CAD build for the part. Positions are in the model's coordinates, mm. A direction names the side the tool comes from. Give positions to 0.01 mm unless a question says otherwise; leave off trailing zeros. Loops run counter-clockwise (first coordinate to the right, second up) from the corner with the lowest first, then second, coordinate; pieces in that order, holes last. Notation, with made-up numbers: (-34.75, -26) - (-19.75, -26) arc R18 cw to (-19.75, 0) - close; hole circle Ø9 at (89.5, -28.75). An arc over 180 degrees is marked (long way). Return JSON: item names as keys, results as strings.
from build123d import *

# Parameters (mm, degrees)
SKETCH_1_R             = 1.55
SKETCH_1_W             = 8
SKETCH_1_H             = 3.5
EXTRUDE_1_DEPTH        = 2
EXTRUDE_START          = 2
EXTRUDE_2_DEPTH        = 2
FILLET_1_R             = 66.25
FILLET_4_R             = 1.5
SKETCH_7093_W          = 3
SKETCH_7093_H          = 15.5
SKETCH_7093_H_2        = 8.5
CUT_EXTRUDE_7585_DEPTH = 243.593574343
SKETCH_4_R             = 1.55
CUT_EXTRUDE_3_DEPTH    = 243.593574343
FILLET_5_R             = 3.5
SKETCH_8290_R          = 0.5
CUT_EXTRUDE_8728_DEPTH = 243.593574343


with BuildPart() as part:
    # 草图1 → 凸台-拉伸1 (new body)
    with BuildSketch(Plane.XY):
        with BuildLine():
            Line((155.184819061, -135.622927906), (110.023968778, -178.814555125))
            Line((110.023968778, -178.814555125), (45.146014647, -178.814555125))
            Line((45.146014647, -178.814555125), (22.125974708, -159.870216287))
            Line((22.125974708, -159.870216287), (-22.125974708, -159.870216287))
            Line((-22.125974708, -159.870216287), (-45.146014647, -178.814555125))
            Line((-45.146014647, -178.814555125), (-110.023968778, -178.814555125))
            Line((-110.023968778, -178.814555125), (-157.725302675, -148.011482983))
            Line((-157.725302675, -148.011482983), (-157.725302675, -39.583555807))
            Line((-157.725302675, -39.583555807), (-163.929854474, -22.461337388))
            Line((-163.929854474, -22.461337388), (-163.929854474, -5.84291361))
            Line((-163.929854474, -5.84291361), (-155.504077083, -3.600927376))
            Line((-155.504077083, -3.600927376), (-155.504077083, -0.25))
            Line((-155.504077083, -0.25), (-135.192862201, -0.25))
            Line((-135.192862201, -0.25), (-135.192862201, -5.85))
            Line((-135.192862201, -5.85), (-129.719705899, -10.576675864))
            Line((-129.719705899, -10.576675864), (-129.719705899, -18.798405758))
            Line((-129.719705899, -18.798405758), (-135.893457817, -19.398277466))
            Line((-135.893457817, -19.398277466), (-141.850432027, -24.52026455))
            Line((-141.850432027, -24.52026455), (-141.850432027, -87.17927527))
            ThreePointArc((-141.850432027, -87.17927527), (-143.273456416, -95.14794796), (-143.75, -103.228644035))
            ThreePointArc((-143.75, -103.228644035), (-106.74521716, -164.210638816), (-35.566620001, -159.54534708))
            Line((-35.566620001, -159.54534708), (-22.125974708, -150.134105928))
            Line((-22.125974708, -150.134105928), (22.125974708, -150.134105928))
            Line((22.125974708, -150.134105928), (35.566620001, -159.54534708))
            ThreePointArc((35.566620001, -159.54534708), (106.74521716, -164.210638816), (143.75, -103.228644035))
            ThreePointArc((143.75, -103.228644035), (143.461588771, -96.937907752), (142.598774895, -90.699951658))
            Line((142.598774895, -90.699951658), (142.966212817, -58.312660923))
            Line((142.966212817, -58.312660923), (131.782009345, -48.416521639))
            Line((131.782009345, -48.416521639), (120.077827626, -48.416521639))
            Line((120.077827626, -48.416521639), (114.577827626, -42.916521639))
            Line((114.577827626, -42.916521639), (114.577827626, -32.685002446))
            ThreePointArc((114.577827626, -32.685002446), (131.61274691, -32.289659724), (148.501080229, -30.024937097))
            ThreePointArc((148.501080229, -30.024937097), (150.418326561, -30.295579056), (151.770912833, -31.681072088))
            Line((151.770912833, -31.681072088), (155.01141709, -38.479630817))
            ThreePointArc((155.01141709, -38.479630817), (155.29338172, -39.526516509), (155.184819061, -40.605260155))
            Line((155.184819061, -40.605260155), (155.184819061, -135.622927906))
        make_face()
        with Locations((-133.806240002, -14.600927376)):
            Circle(SKETCH_1_R, mode=Mode.SUBTRACT)
        with Locations((120.182300402, -39.335)):
            Circle(SKETCH_1_R, mode=Mode.SUBTRACT)
        with Locations((149.25, -76.25)):
            Rectangle(SKETCH_1_W, SKETCH_1_H, mode=Mode.SUBTRACT)
        with Locations((-149.25, -76.25)):
            Rectangle(SKETCH_1_W, SKETCH_1_H, mode=Mode.SUBTRACT)
    extrude(amount=EXTRUDE_1_DEPTH)

    # 草图2 → 凸台-拉伸2 (add)
    with BuildSketch(Plane.XY.offset(EXTRUDE_START)):
        Polygon((155.184819061, -68.75), (158.934819061, -70.915063509), (158.934819061, -81.584936491), (155.184819061, -83.75), align=None)
        Polygon((-157.725302675, -68.75), (-157.725302675, -83.75), (-162.225302675, -81.886038969), (-162.225302675, -70.613961031), align=None)
    extrude(amount=-EXTRUDE_2_DEPTH)

    # 圆角1
    fillet_1_edges = [part.edges().sort_by_distance(p)[0] for p in [
        (-141.850432027, -87.17927527, 1),
        (142.598774895, -90.699951658, 1),
    ]]
    fillet(fillet_1_edges, radius=FILLET_1_R)

    # 圆角4
    fillet_4_edges = [part.edges().sort_by_distance(p)[0] for p in [
        (158.934819061, -81.584936491, 1),
        (158.934819061, -70.915063509, 1),
        (155.184819061, -68.75, 1),
        (155.184819061, -83.75, 1),
        (-162.225302675, -70.613961031, 1),
        (-162.225302675, -81.886038969, 1),
        (-157.725302675, -83.75, 1),
        (-157.725302675, -68.75, 1),
        (-155.504077083, -0.25, 1),
    ]]
    fillet(fillet_4_edges, radius=FILLET_4_R)

    # Sketch 7093 → Cut-Extrude 7585 (cut, through all)
    with BuildSketch(Plane.XY.offset(2)):
        with Locations((-149.5, -98.25)):
            Rectangle(SKETCH_7093_W, SKETCH_7093_H)
        with Locations((-149.5, -55.25)):
            Rectangle(SKETCH_7093_W, SKETCH_7093_H_2)
        Polygon((-134.649663794, -153.091956536), (-124.148766338, -159.87289693), (-125.776192033, -162.39311232), (-136.277089488, -155.612171926), align=None)
    extrude(amount=-CUT_EXTRUDE_7585_DEPTH, mode=Mode.SUBTRACT)

    # 草图4 → 切除-拉伸3 (cut, through all)
    with BuildSketch(Plane.XY):
        with Locations((-142.225302675, -140.821536198)):
            Circle(SKETCH_4_R)
        with Locations((-45.146014647, -171.064555125)):
            Circle(SKETCH_4_R)
        with Locations((-106.712983856, -171.314555125)):
            Circle(SKETCH_4_R)
        with Locations((46.656002152, -172.314555125)):
            Circle(SKETCH_4_R)
        with Locations((145.684819061, -132.301036976)):
            Circle(SKETCH_4_R)
    extrude(amount=CUT_EXTRUDE_3_DEPTH, mode=Mode.SUBTRACT)

    # 圆角5
    fillet_5_edges = [part.edges().sort_by_distance(p)[0] for p in [
        (-135.192862201, -5.85, 1),
        (-129.719705899, -10.576675864, 1),
        (-129.719705899, -18.798405758, 1),
        (-135.893457817, -19.398277466, 1),
        (-141.850432027, -24.52026455, 1),
        (131.782009345, -48.416521639, 1),
        (114.577827626, -32.685002446, 1),
    ]]
    fillet(fillet_5_edges, radius=FILLET_5_R)

    # Sketch 8290 → Cut-Extrude 8728 (cut, through all)
    with BuildSketch(Plane.XY):
        with Locations((-151, -51)):
            Circle(SKETCH_8290_R)
        with Locations((-148, -51)):
            Circle(SKETCH_8290_R)
        with Locations((-151, -59.5)):
            Circle(SKETCH_8290_R)
        with Locations((-148, -59.5)):
            Circle(SKETCH_8290_R)
        with Locations((-153.25, -74.5)):
            Circle(SKETCH_8290_R)
        with Locations((-145.25, -74.5)):
            Circle(SKETCH_8290_R)
        with Locations((-145.25, -78)):
            Circle(SKETCH_8290_R)
        with Locations((-153.25, -78)):
            Circle(SKETCH_8290_R)
        with Locations((-151, -90.5)):
            Circle(SKETCH_8290_R)
        with Locations((-148, -90.5)):
            Circle(SKETCH_8290_R)
        with Locations((-151, -106)):
            Circle(SKETCH_8290_R)
        with Locations((-148, -106)):
            Circle(SKETCH_8290_R)
        with Locations((-134.649663794, -153.091956536)):
            Circle(SKETCH_8290_R)
        with Locations((-136.277089488, -155.612171926)):
            Circle(SKETCH_8290_R)
        with Locations((-124.148766338, -159.87289693)):
            Circle(SKETCH_8290_R)
        with Locations((-125.776192033, -162.39311232)):
            Circle(SKETCH_8290_R)
        with Locations((145.25, -74.5)):
            Circle(SKETCH_8290_R)
        with Locations((153.25, -74.5)):
            Circle(SKETCH_8290_R)
        with Locations((153.25, -78)):
            Circle(SKETCH_8290_R)
        with Locations((145.25, -78)):
            Circle(SKETCH_8290_R)
    extrude(amount=CUT_EXTRUDE_8728_DEPTH, mode=Mode.SUBTRACT)


solid = part.part
1. Drill centre lines: probe 1 along X at (y, z) = (-105, 0.45); probe 2 along X at (y, z) = (-94, 0.15); probe 3 along X at (y, z) = (-61, 0.9). Where is each one in solid material? Low to high.
Values follow:
{"probe 1": "x = -157.73 to -151, -148 to -143.73, 143.73 to 155.18", "probe 2": "x = -157.73 to -151, -148 to -143.13, 143.13 to 155.18", "probe 3": "x = -157.73 to -141.85, 142.94 to 155.18"}
2. Drop flat-ended pins along their axis: P1, Ø1, axis at y = -81, z = 1.5, coming from the -X side; P2, Ø0.6, axis at x = 148, z = 0.5, coming from the -Y side; P3, Ø1, axis at x = 7, z = 1, coming from the -Y side. Give the stop position or say it passes through.
Values follow:
{"P1": "stops at x = -162.23", "P2": "stops at y = -142.78", "P3": "stops at y = -159.87"}
3. Pull direction Y, two halves, no side cores. Call faces 5 (the face through (-26, -155, 2)), 6 (the face through (137.942, -53.867, 0.986)), 7 (the face through (28.75, -154.77, 0.99)), 8 (the face through (-130.959, -159.046, 1.014)): +Y half, -Y half, draft (parallel to the pull), parting line (faces both ways), or undercut.
Values follow:
{"face 5": "draft", "face 6": "undercut", "face 7": "+Y half", "face 8": "undercut"}
4. Which spindle directions (+Z, -Z, +X, -X, +Y, -Y) get a long thin tool onto all of the face, cutting with end or side? Do faces 1 (the face through (-160.8, -31.1, 1)), 2 (the face through (-129.467, -156.439, 1.014)), 3 (the face through (33.797, -169.475, 0.986)), 4 (the face through (-28.94, -154.906, 0.986)). Say none if no direction does.
Values follow:
{"face 1": "+Z, -Z, -X", "face 2": "+Z, -Z", "face 3": "+Z, -Z, -Y", "face 4": "+Z, -Z, +Y"}
5. Cut at D-D, the plane x = 13. Write the cut outline in (y, z), plus the area to 3 significant figures.
Values follow:
{"outline": "(-159.87, 0) - (-150.13, 0) - (-150.13, 2) - (-159.87, 2) - close", "area": "19.5 mm²"}
6. Cut at C-C, the plane z = 0.8. Give the number of separate pieces and of enclosed holes in the cut face, plus the area to 3 significant figures.
Values follow:
{"separate pieces": "1", "enclosed holes": "12", "area": "7,880 mm²"}
7. Cut at A-A, the plane x = 139. Write the cut outline in (y, z).
Values follow:
{"outline": "(-151.1, 0) - (-128.34, 0) - (-128.34, 2) - (-151.1, 2) - close; (-54.8, 0) - (-31.53, 0) - (-31.53, 2) - (-54.8, 2) - close"}
8. Cut at B-B, the plane y = -112. Write the cut outline in (x, z), plus the area to 3 significant figures.
Values follow:
{"outline": "(-157.73, 0) - (-143.19, 0) - (-143.19, 2) - (-157.73, 2) - close; (143.19, 0) - (155.18, 0) - (155.18, 2) - (143.19, 2) - close", "area": "53.1 mm²"}
